Verification items for the finished model (mm, model axes). Coordinates: 2 decimals unless noted, no trailing zeros. Order: outer loops, then holes, each group sorted by start corner. A loop starts at its lowest first (then second) coordinate and runs counter-clockwise, first axis right, second up. Notation, with made-up numbers: (53, -6.75) -> (86, -6.75) arc R24 ccw to (86, 31.25) -> close; hole circle Ø6 at (3, -37). An arc over 180 degrees is marked (long way). Use CSV: the item, a comma, the result in double quotes. Start each with the question number.
1) Scan lines: line 1 along Y through (x, z) = (-1.3, -1.7); line 2 along X through (y, z) = (9, 2.15); line 3 along X through (y, z) = (8.75, 0.5). Record each from-to range of solid material in increasing order.
2) Go/stop test with a flat-tipped pin: pin 1 (1 mm diameter, centred on x = -1.5, y = 5, fed in from +Z). Record where the tip stops, or that it passes through.
3) Sectioned sample at A-A on y = 8. Record the boundary of the cut face in (x, z), then the cut area to 3 significant figures.
from build123d import *

# Parameters (mm, degrees)
SKETCH1_R           = 2.6
BOSS_EXTRUDE1_DEPTH = 15
CHAMFER1_SIZE       = 0.8
SKETCH2_R           = 2.6
SKETCH2_R_2         = 2.5
CUT_EXTRUDE2_DEPTH  = 16.444092722


with BuildPart() as part:
    # Sketch1 → Boss-Extrude1 (new body)
    with BuildSketch(Plane(origin=(0, 0, 0), x_dir=(1, 0, 0), z_dir=(0, 1, 0))):
        with Locations(Location((0, 0, 0), (0, 0, 270))):
            Circle(SKETCH1_R)
    extrude(amount=BOSS_EXTRUDE1_DEPTH)

    # Chamfer1
    chamfer1_edges = [part.edges().sort_by_distance(p)[0] for p in [
        (0, 0, -2.6),
        (0, 15, -2.6),
    ]]
    chamfer(chamfer1_edges, length=CHAMFER1_SIZE)

    # Sketch2 → Cut-Extrude2 (cut, through all)
    with BuildSketch(Plane(origin=(0, 15, 0), x_dir=(1, 0, 0), z_dir=(0, 1, 0))):
        Circle(SKETCH2_R)
        with Locations(Location((0, 0, 0), (0, 0, 270))):
            Circle(SKETCH2_R_2, mode=Mode.SUBTRACT)
    extrude(amount=-CUT_EXTRUDE2_DEPTH, mode=Mode.SUBTRACT)


solid = part.part
Answers follow:
1,line 1,"y = 0.34 to 14.66"
1,line 2,"x = -1.28 to 1.28"
1,line 3,"x = -2.45 to 2.45"
2,pin 1,"stops at z = 2.29"
3,outline,"circle Ø5 at (0, 0)"
3,area,"19.6 mm²"
